Can you work these out from the model? Positions are in its coordinate system, mm. Face numbers are marked on the shaded views. Give positions to 0.01 mm unless a question says otherwise; leave off trailing zeros. Write each loop counter-clockwise with the first axis right and the second up, starting at its lowest first coordinate (ties: lowest second). Pieces come first, ordered by that corner, then holes. Notation, with made-up numbers: (88, 49) - (97, 49) arc R19 ccw to (97, 66) - close; hole circle Ø4 at (30, -34.5). An arc over 180 degrees is marked (long way). Return JSON: item names as keys, results as strings. Group by question number.
from build123d import *

# Parameters (mm, degrees)
F0_R     = 8.89
F1_DEPTH = 25.4
F1_TAPER = 2
F2_T     = -0.508
F3_R     = 0.508


with BuildPart() as f1:
    # F0 (on Top) → F1 (new body)
    with BuildSketch(Plane.XY):
        Circle(F0_R)
    extrude(amount=F1_DEPTH, taper=F1_TAPER)

    # F2
    f2_openings = [f1.faces().sort_by_distance(p)[0] for p in [
        (0, 0, 0),
    ]]
    offset(amount=F2_T, openings=f2_openings)

    # F3
    f3_edges = [f1.edges().sort_by_distance(p)[0] for p in [
        (-8.003012, 0, 25.4),
    ]]
    fillet(f3_edges, radius=F3_R)


solid = f1.part
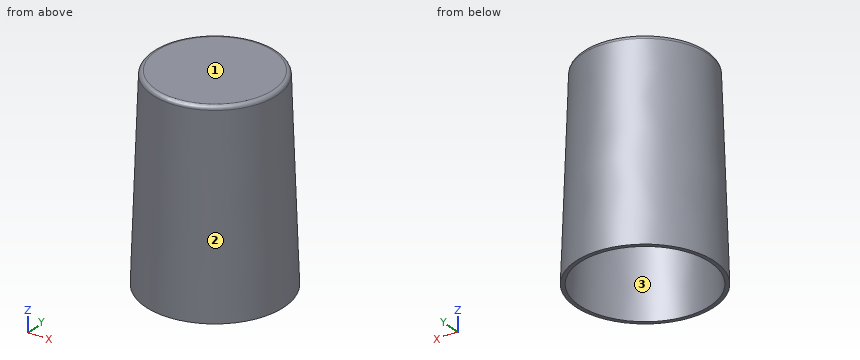
1) Imagine slicing it at A-A, the plane x = 0. Write out the boundary of the cut face in (y, z), and give its area (3 significant figures).
2) I need wall thicknesses on line 1 along Z through (x, y) = (5, -3); line 2 along Y through (x, z) = (-2, 12.5); line 3 along Y through (x, z) = (7.5, 7.5). Which ranges of each line are inside material? Lowest first, please.
3) Imagine slicing it at C-C, the plane z = 3.25. Write out the boundary of the cut face in (x, y).
4) Will these pins go through, and if not, where does the flat tip stop? pin 1 Ø3 at (y, z) = (2, 15) entering from -X; pin 2 Ø5 at (x, z) = (-0.5, 9.5) entering from +Y; pin 3 Ø1 at (y, z) = (2.5, 17.5) entering from +X.
5) We'd pull the mould along X, two halves only. Please class the marked faces 1, 2 and 3: pulls with the +X half, pulls with the -X half, needs draft (parallel to the pull), parting line crosses it, or undercut.
6) Imagine slicing it at D-D, the plane z = 9. Write out the boundary of the cut face in (x, y), and give its area (3 significant figures).
Resolved:
{
 "1": {"outline": "(-8.89, 0) - (-8.38, 0) - (-7.51, 24.89) - (7.51, 24.89) - (8.38, 0) - (8.89, 0) - (8.02, 24.91) arc R0.51 ccw to (7.51, 25.4) - (-7.51, 25.4) arc R0.51 ccw to (-8.02, 24.91) - close", "area": "33.3 mm^2"},
 "2": {"line 1": "24.89 to 25.4", "line 2": "-8.21 to -7.69, 7.69 to 8.21", "line 3": "-4.27 to -3.11, 3.11 to 4.27"},
 "3": {"outline": "circle Ø17.55 at (0, 0); hole circle Ø16.54 at (0, 0)"},
 "4": {"pin 1": "x = -8.36", "pin 2": "y = 8.64", "pin 3": "x = 8.03"},
 "5": {"face 1": "needs draft", "face 2": "parting line crosses it", "face 3": "undercut"},
 "6": {"outline": "circle Ø17.15 at (0, 0); hole circle Ø16.13 at (0, 0)", "area": "26.6 mm^2"}
}
